The model under review builds one solid part; all positions refer to its coordinate system, in mm. A direction names the side the tool comes from. Round coordinates to 2 decimals unless told otherwise and drop trailing zeros. Write each loop counter-clockwise with the first axis right and the second up, starting at its lowest first coordinate (ties: lowest second). Pieces come first, ordered by that corner, then holes. Notation, with made-up numbers: (81.5, -22) -> (129.5, -22) arc R13 cw to (129.5, -6) -> close; hole circle Ø10 at (62.5, 84). An arc over 180 degrees is marked (long way). Return JSON: item names as keys, results as strings. Group by question number.
1. Tool access review of faces 4 (the flat face through (0, 1, -2)), 5 (the conical face through (1.466, -1.268, -1.779)): name each direction out of +Z, -Z, +X, -X, +Y, -Y from which nothing blocks a thin tool from reaching the whole face with its end or side.
2. Mouldability with a two-part tool opening along X and no side actions: class faces 1 (the flat face through (22, 1, -2)), 2 (the flat face through (10.8, 1.5, -2)), 3 (the conical face through (19.449, -1.268, -2.174)) as pulls with the +X half, pulls with the -X half, needs draft (parallel to the pull), parting line crosses it, or undercut.
3. Take a section at C-C, the plane x = 9.5. Write out the cut boundary in (y, z).
4. Take a section at A-A, the plane x = 13. Write out the cut boundary in (y, z).
5. Clearance check with flat-ended pins moving along their axes: P1, Ø1.2, axis at x = 7, z = -2.5, coming from the -Y side; P2, Ø1.5, axis at y = -1.5, z = -0.5, coming from the +X side (3 decimals). State where each tip first meets the part, or that it passes through.
6. Take a section at B-B, the plane y = 1.15. Give the number of separate pieces and of enclosed holes in the cut face, then the cut area to 3 significant figures.
7. Take a section at D-D, the plane y = -1.5. Write out the cut boundary in (x, z), then the cut area to 3 significant figures.
8. For line 1 along Y through (x, z) = (4, -3.6); line 2 along X through (y, z) = (-1.5, -1.6); line 3 along X through (y, z) = (-0.6, -2.25), list the stretches that pass through material, from the lowest coordinate up. Write a range as from..to.
from build123d import *

# Parameters (mm, degrees)
SKETCH1_W           = 22
SKETCH1_H           = 4
BOSS_EXTRUDE1_DEPTH = 1.5
SKETCH2_W           = 0.5
SKETCH2_H           = 0.5
CUT_EXTRUDE1_DEPTH  = 2
SKETCH3_R           = 0.01
CUT_EXTRUDE2_DEPTH  = 1.5
SKETCH4_R           = 0.6
BOSS_EXTRUDE2_DEPTH = 2.5
BOSS_EXTRUDE2_TAPER = 1


with BuildPart() as part:
    # Sketch1 → Boss-Extrude1 (new body)
    with BuildSketch(Plane(origin=(0, 0, 0), x_dir=(1, 0, 0), z_dir=(0, 1, 0))):
        with Locations((11, 2)):
            Rectangle(SKETCH1_W, SKETCH1_H)
    extrude(amount=BOSS_EXTRUDE1_DEPTH)

    # Sketch2 → Cut-Extrude1 (cut)
    with BuildSketch(Plane(origin=(0, 1.5, 0), x_dir=(1, 0, 0), z_dir=(0, 1, 0))):
        with Locations((3, 3)):
            Rectangle(SKETCH2_W, SKETCH2_H)
        with Locations((1, 3)):
            Rectangle(SKETCH2_W, SKETCH2_H)
        with Locations((5, 3)):
            Rectangle(SKETCH2_W, SKETCH2_H)
        with Locations((7, 3)):
            Rectangle(SKETCH2_W, SKETCH2_H)
        with Locations((9, 3)):
            Rectangle(SKETCH2_W, SKETCH2_H)
        with Locations((11, 3)):
            Rectangle(SKETCH2_W, SKETCH2_H)
        with Locations((13, 3)):
            Rectangle(SKETCH2_W, SKETCH2_H)
        with Locations((15, 3)):
            Rectangle(SKETCH2_W, SKETCH2_H)
        with Locations((17, 3)):
            Rectangle(SKETCH2_W, SKETCH2_H)
        with Locations((19, 3)):
            Rectangle(SKETCH2_W, SKETCH2_H)
        with Locations((21, 3)):
            Rectangle(SKETCH2_W, SKETCH2_H)
        with Locations((1, 1)):
            Rectangle(SKETCH2_W, SKETCH2_H)
        with Locations((3, 1)):
            Rectangle(SKETCH2_W, SKETCH2_H)
        with Locations((5, 1)):
            Rectangle(SKETCH2_W, SKETCH2_H)
        with Locations((7, 1)):
            Rectangle(SKETCH2_W, SKETCH2_H)
        with Locations((9, 1)):
            Rectangle(SKETCH2_W, SKETCH2_H)
        with Locations((11, 1)):
            Rectangle(SKETCH2_W, SKETCH2_H)
        with Locations((13, 1)):
            Rectangle(SKETCH2_W, SKETCH2_H)
        with Locations((15, 1)):
            Rectangle(SKETCH2_W, SKETCH2_H)
        with Locations((17, 1)):
            Rectangle(SKETCH2_W, SKETCH2_H)
        with Locations((19, 1)):
            Rectangle(SKETCH2_W, SKETCH2_H)
        with Locations((21, 1)):
            Rectangle(SKETCH2_W, SKETCH2_H)
    extrude(amount=-CUT_EXTRUDE1_DEPTH, mode=Mode.SUBTRACT)

    # Sketch3 → Cut-Extrude2 (cut)
    with BuildSketch(Plane(origin=(0, 1.5, 0), x_dir=(1, 0, 0), z_dir=(0, 1, 0))):
        with Locations((11, 2)):
            Circle(SKETCH3_R)
    extrude(amount=-CUT_EXTRUDE2_DEPTH, mode=Mode.SUBTRACT)

    # Sketch4 → Boss-Extrude2 (add)
    with BuildSketch(Plane(origin=(0, 0, 0), x_dir=(-1, 0, 0), z_dir=(0, -1, 0))):
        with Locations((-20, 2)):
            Circle(SKETCH4_R)
        with Locations((-2, 2)):
            Circle(SKETCH4_R)
    extrude(amount=BOSS_EXTRUDE2_DEPTH, taper=BOSS_EXTRUDE2_TAPER)


solid = part.part
Output:
{
 "1": {"face 4": "+Z, -Z, -X, +Y, -Y", "face 5": "-Y"},
 "2": {"face 1": "pulls with the +X half", "face 2": "needs draft", "face 3": "undercut"},
 "3": {"outline": "(0, -4) -> (1.5, -4) -> (1.5, 0) -> (0, 0) -> close"},
 "4": {"outline": "(0, -4) -> (1.5, -4) -> (1.5, -3.25) -> (0, -3.25) -> close; (0, -2.75) -> (1.5, -2.75) -> (1.5, -1.25) -> (0, -1.25) -> close; (0, -0.75) -> (1.5, -0.75) -> (1.5, 0) -> (0, 0) -> close"},
 "5": {"P1": "stops at y = 0", "P2": "passes through"},
 "6": {"separate pieces": "1", "enclosed holes": "23", "area": "82.5 mm^2"},
 "7": {"outline": "circle Ø1.15 at (2, -2); circle Ø1.15 at (20, -2)", "area": "2.07 mm^2"},
 "8": {"line 1": "y = 0..1.5", "line 2": "x = 1.59..2.41, 19.59..20.41", "line 3": "x = 1.47..2.53, 19.47..20.53"}
}
